```python
from build123d import *

# Parameters (mm, degrees)
SKETCH_1_R      = 15
SKETCH_1_R_2    = 7.5
EXTRUDE_1_DEPTH = 52.5
SKETCH_2_R      = 12.5
EXTRUDE_2_DEPTH = 5
FILLET_1_R      = 4
FILLET_2_R      = 20
FILLET_3_R      = 2


with BuildPart() as part:
    # 스케치1 → 보스-돌출1 (new, symmetric)
    with BuildSketch(Plane(origin=(0, 0, 0), x_dir=(0, 0, -1), z_dir=(1, 0, 0))):
        Circle(SKETCH_1_R)
        Circle(SKETCH_1_R_2, mode=Mode.SUBTRACT)
    extrude(amount=EXTRUDE_1_DEPTH, both=True)

    # 스케치2 → 보스-돌출2 (add, symmetric)
    with BuildSketch(Plane(origin=(0, 0, 0), x_dir=(1, 0, 0), z_dir=(0, 1, 0))):
        with BuildLine():
            Line((-47.5, -12), (-47.5, -240))
            ThreePointArc((-47.5, -240), (-22.5, -265), (2.5, -240))
            Line((2.5, -240), (2.5, -215))
            Line((2.5, -215), (47.5, -60))
            Line((47.5, -60), (47.5, -12))
            Line((47.5, -12), (22.5, -12))
            Line((22.5, -12), (22.5, -23))
            Line((22.5, -23), (-22.5, -23))
            Line((-22.5, -23), (-22.5, -12))
            Line((-22.5, -12), (-47.5, -12))
        make_face()
        with Locations(Location((-22.5, -240, 0), (0, 0, 270))):
            Circle(SKETCH_2_R, mode=Mode.SUBTRACT)
        with BuildLine():
            Line((-14.658615093, -184.435160923), (22.5, -56.444375602))
            Line((22.5, -56.444375602), (22.5, -48))
            Line((22.5, -48), (-22.5, -48))
            Line((-22.5, -48), (-22.5, -183.319920143))
            ThreePointArc((-22.5, -183.319920143), (-19.063231911, -187.280067844), (-14.658615093, -184.435160923))
        make_face(mode=Mode.SUBTRACT)
    extrude(amount=EXTRUDE_2_DEPTH, both=True)

    # 필렛1
    fillet_1_edges = [part.edges().sort_by_distance(p)[0] for p in [
        (22.5, 0, 23),
        (-22.5, 0, 23),
        (22.5, 0, 48),
        (-22.5, 0, 48),
        (22.5, 0, 56.444375602),
    ]]
    fillet(fillet_1_edges, radius=FILLET_1_R)

    # 필렛2
    fillet_2_edges = [part.edges().sort_by_distance(p)[0] for p in [
        (47.5, 0, 60),
    ]]
    fillet(fillet_2_edges, radius=FILLET_2_R)

    # 필렛3
    fillet_3_edges = [part.edges().sort_by_distance(p)[0] for p in [
        (-47.5, 0, 15),
        (-35, -5, 14.142135624),
        (-35, 5, 14.142135624),
        (-22.5, 0, 15),
        (22.5, 0, 15),
        (35, -5, 14.142135624),
        (35, 5, 14.142135624),
        (47.5, 0, 15),
    ]]
    fillet(fillet_3_edges, radius=FILLET_3_R)


solid = part.part
```
The listing builds one solid part. Answer for the finished solid, in the listing's coordinates (mm). A direction names the side the tool comes from. Coordinates: 2 decimals unless noted, no trailing zeros. Write each loop counter-clockwise with the first axis right and the second up, starting at its lowest first coordinate (ties: lowest second). Pieces come first, ordered by that corner, then holes. Notation, with made-up numbers: (45, 23) - (63, 23) arc R28 cw to (63, 51) - close; hole circle Ø6 at (4, 83). An arc over 180 degrees is marked (long way). Return JSON: item names as keys, results as strings. Group by question number.
Q1. For a pull along X with two mould halves and no side action, classify faces 6 (the flat face through (24.294, 0.07, 139.932)), 7 (the flat face through (0, 0, 23)), 8 (the flat face through (-52.5, 7, 4)) as +X half, -X half, draft (parallel to the pull), parting line (faces both ways), or undercut.
Q2. The part is cut by section A-A on y = 0. State how many separate pieces and enclosed holes the cut face has, and give its area (3 significant figures).
Q3. Which of the six approach directions +Z, -Z, +X, -X, +Y, -Y give full straight-line access (tool end or side, diameter ignored) to faces 1 (the flat face through (2.5, 0, 228)), 2 (the flat face through (-1, 5, 138)), 3 (the flat face through (0, 0, 48)), 4 (the flat face through (-1, -5, 138)), 5 (the flat face through (-47.5, 0, 127))?
Q4. The part is cut by section B-B on z = 0. Write down the section's boundary in (x, y), and give its area (4 significant figures).
Q5. Find the intervals of material crossed by line 1 along Y through (x, z) = (-14, 0); line 2 along X through (y, z) = (-0.75, 240); line 3 along Y through (x, z) = (38, 48), in increasing order. Write a range as [from, to].
Q6. The part is cut by section D-D on x = 5. Write down the section's boundary in (y, z).
Q7. The part is cut by section C-C on x = -26. Write down the section's boundary in (y, z).
Q8. Flat-ended cylindrical pins translate along their axes: pin 1 Ø5 at (y, z) = (1, 226) entering from +X; pin 2 Ø11 at (y, z) = (-2, 92.5) entering from +X; pin 3 Ø8 at (x, y) = (-36, -9) entering from -Z; pin 4 Ø5 at (x, y) = (3, -1.5) entering from -Z. Find the tip coordinate at first contact, or state that the pin passes through.
Evaluation:
{
 "1": {"face 6": "+X half", "face 7": "undercut", "face 8": "-X half"},
 "2": {"separate pieces": "2", "enclosed holes": "3", "area": "14,700 mm2"},
 "3": {"face 1": "+Z, +X, +Y, -Y", "face 2": "+Z, +X, -X, +Y", "face 3": "+Y, -Y", "face 4": "+Z, +X, -X, -Y", "face 5": "+Z, -X, +Y, -Y"},
 "4": {"outline": "(-52.5, -15) - (52.5, -15) - (52.5, -7.5) - (-52.5, -7.5) - close; (-52.5, 7.5) - (52.5, 7.5) - (52.5, 15) - (-52.5, 15) - close", "area": "1,575 mm2"},
 "5": {"line 1": "y = [-15, -7.5], [7.5, 15]", "line 2": "x = [-47.5, -35], [-10, 2.5]", "line 3": "y = [-5, 5]"},
 "6": {"outline": "circle Ø30 at (0, 0); (-5, 23) - (5, 23) - (5, 48) - (-5, 48) - close; (-5, 116.72) - (5, 116.72) - (5, 206.39) - (-5, 206.39) - close; hole circle Ø15 at (0, 0)"},
 "7": {"outline": "(-6.18, 13.67) arc R15 ccw (long way) to (6.18, 13.67) arc R2 cw to (5, 15.49) - (5, 228) - (-5, 228) - (-5, 15.49) arc R2 cw to start; (-5, 252) - (5, 252) - (5, 264.75) - (-5, 264.75) - close; hole circle Ø15 at (0, 0)"},
 "8": {"pin 1": "stops at x = 2.5", "pin 2": "stops at x = 39.66", "pin 3": "stops at z = -14.14", "pin 4": "stops at z = -15"}
}
